Autodesk Inventor part; units mm, degrees
ref_plane "YZ Plane" through (0, 0, 0) normal (1, 0, 0) x (0, 1, 0)
ref_plane "XZ Plane" through (0, 0, 0) normal (0, 1, 0) x (-1, 0, 0)
ref_plane "XY Plane" through (0, 0, 0) normal (0, 0, 1) x (1, 0, 0)
sketch "Sketch1" plane through (0, 0, 0) normal (1, 0, 0) x (0, 1, 0)
  line L0 (0, 0) -> (20.7, 0)
  line L1 (20.7, 0) -> (20.7, -45.6)
  line L2 (20.7, -45.6) -> (0, -45.6)
  line L3 (0, -45.6) -> (0, 0)
  circle A0 centre (10.35, -9.5) radius 8
  circle A1 centre (10.35, -35.5) radius 8
  line L4 (21.7, -46.6) -> (21.7, 1)
  line L5 (21.7, 1) -> (-1, 1)
  line L6 (-1, 1) -> (-1, -46.6)
  line L7 (-1, -46.6) -> (21.7, -46.6)
  dimension "Breite" = 20.7
  dimension "Länge" = 45.6
  dimension "Kreise1" = 16
  dimension "BreiteBisKreise1" = 9.5
  dimension "LangeBisKreise" = 10.35
  dimension "KreiseCenter1BisKreiseCenter2" = 26
  dimension "Kreise2" = 16
  dimension "LangeBisKreise2" = 10.35
  dimension "d14" = 1
extrude "Extrusion1" add sketch "Sketch1" along normal blind 15 contours L0 L1 L2 L3 | A0 | A1
extrude "Extrusion2" add sketch "Sketch1" along normal up to surface (15 mm away) contours L7 L6 L5 L4
sketch "Sketch2" plane through (15, 0, 0) normal (1, 0, 0) x (0, 0, -1)
  line L0 (0, 20.7) -> (45.6, 20.7)
  line L1 (56.12, 0) -> (-10.52, 0)
  line L2 (45.6, 20.7) -> (45.6, 0)
  line L3 (0, -5.54) -> (0, 26.24)
  line L4 (0, 20.7) -> (45.6, 20.7)
  line L5 (45.6, 20.7) -> (45.6, 0)
  line L6 (45.6, 0) -> (0, 0)
  line L7 (0, 0) -> (0, 20.7)
extrude "Extrusion3" cut sketch "Sketch2" against normal blind 13
extrude "Extrusion4" cut sketch "Sketch1" along normal blind 11 contours A0 | A1
sketch "Sketch3" plane through (15, 0, 0) normal (1, 0, 0) x (0, 0, -1)
  line L0 (45.6, 20.7) -> (45.6, 0)
  line L1 (45.6, 0) -> (0, 0)
  line L2 (0, 0) -> (0, 20.7)
  line L3 (0, 20.7) -> (45.6, 20.7)
  line L4 (-1, 21.7) -> (46.6, 21.7)
  line L5 (-1, -1) -> (-1, 21.7)
  line L6 (46.6, -1) -> (-1, -1)
  line L7 (46.6, 21.7) -> (46.6, -1)
  line L8 (0, 0) -> (0, 20.7)
  line L9 (0, 0) -> (16.5, 0)
  line L10 (45.6, 0) -> (0, 0)
  line L11 (45.6, 20.7) -> (45.6, 0)
  line L12 (45.6, 0) -> (29.1, 0)
  line L13 (-1, -1) -> (46.6, -1)
  line L14 (16.5, -1) -> (16.5, -10.5)
  line L15 (29.1, -1) -> (29.1, -10.5)
  line L16 (16.5, -10.5) -> (29.1, -10.5)
  dimension "d21" = 16.5
  dimension "d22" = 16.5
  dimension "d23" = 9.5
  dimension "d24" = 1
  dimension "d26" = 12.6
extrude "Extrusion5" add sketch "Sketch3" against normal blind 4 contours L6 L15 L16 L14
sketch "Sketch4" plane through (15, 0, 0) normal (1, 0, 0) x (0, 0, -1)
  line L0 (45.6, 20.7) -> (45.6, 0)
  line L1 (45.6, 0) -> (0, 0)
  line L2 (0, 0) -> (0, 20.7)
  line L3 (0, 20.7) -> (45.6, 20.7)
  line L4 (-1, 21.7) -> (46.6, 21.7)
  line L5 (-1, -1) -> (-1, 21.7)
  line L6 (16.5, -1) -> (-1, -1)
  line L7 (16.5, -1) -> (16.5, -10.5)
  line L8 (16.5, -10.5) -> (29.1, -10.5)
  line L9 (29.1, -10.5) -> (29.1, -1)
  line L10 (46.6, -1) -> (29.1, -1)
  line L11 (46.6, 21.7) -> (46.6, -1)
  line L12 (29.1, -10.5) -> (29.1, -1)
  line L13 (29.1, -10.5) -> (16.5, -10.5)
  line L14 (29.1, -1) -> (16.5, -1)
  line L15 (16.5, -1) -> (16.5, -10.5)
  line L16 (16.5, -10.5) -> (29.1, -10.5)
  line L17 (29.1, -10.5) -> (29.1, -1)
  line L18 (17, -1.5) -> (28.6, -1.5)
  line L19 (28.6, -1.5) -> (28.6, -10)
  line L20 (28.6, -10) -> (17, -10)
  line L21 (17, -10) -> (17, -1.5)
  line L22 (17, -1.5) -> (17, 0)
  line L23 (45.6, 0) -> (0, 0)
  line L24 (28.6, -1.5) -> (28.6, 0)
  line L25 (17, 0) -> (28.6, 0)
  line L26 (17, -10) -> (17, -10.5)
  line L27 (28.6, -10) -> (28.6, -10.5)
  dimension "d29" = 0.5
extrude "Extrusion6" cut sketch "Sketch4" against normal blind 1 contours L24 L14 L22 L1 | L24 L18 L22 L14 | L19 L20 L21 L18 | L27 L8 L26 L20
fillet "Fillet1" radius 2 2 edges at (13, -1, -29.1) (13, -1, -16.5)
fillet "Fillet2" radius 2 4 edges at (7.5, -1, 1) (7.5, -1, -46.6) (7.5, 21.7, -46.6) (7.5, 21.7, 1)
fillet "Fillet3" radius 1 1 edges at (14, -10.5, -22.8)
fillet "Fillet4" radius 1 2 edges at (13, -10.5, -29.1) (13, -10.5, -16.5)
properties part number "Ultaschal Sensor Gehäuse"
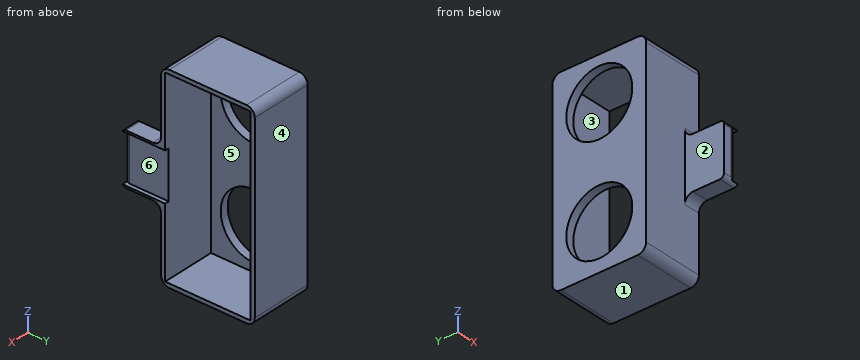
Geometry: final body of the model. Coordinates: model frame, mm. Face numbers are marked on the shaded views. A direction names the side the tool comes from. Give positions to 0.01 mm unless a question says otherwise; leave off trailing zeros. Write each loop counter-clockwise with the first axis right and the second up, starting at its lowest first coordinate (ties: lowest second). Pieces come first, ordered by that corner, then holes. Notation, with made-up numbers: (-26.75, 32) -> (32.25, 32) arc R25 cw to (32.25, 64) -> close; hole circle Ø10 at (22.5, -37.5). An arc over 180 degrees is marked (long way). Answer in a Markdown table with one row per item.
(1) Ray query, line 1 along Z through (x, y) = (1.15, 10.35); line 2 along Y through (x, z) = (0.6, -9.5); line 3 along Z through (x, y) = (13.75, 13.5). Return the intervals inside material, ascending. Write a range as [from, to].
Answers below:
| item | result |
|---|---|
| line 1 | [-46.6, -43.5], [-27.5, -17.5], [-1.5, 1] |
| line 2 | [-1, 2.35], [18.35, 21.7] |
| line 3 | [-46.6, -45.6], [0, 1] |
(2) Section query C-C on x = 10.25. Return loops of the section in (y, z), then the cut area to 3 significant figures.
Answers below:
| item | result |
|---|---|
| outline | (-1, -44.6) arc R2 ccw to (1, -46.6) -> (19.7, -46.6) arc R2 ccw to (21.7, -44.6) -> (21.7, -1) arc R2 ccw to (19.7, 1) -> (1, 1) arc R2 ccw to (-1, -1) -> close; hole (0, -45.6) -> (20.7, -45.6) -> (20.7, 0) -> (0, 0) -> close |
| area | 133 mm^2 |
(3) Section query A-A on z = -35.5. Return loops of the section in (x, y), then the cut area to 3 significant figures.
Answers below:
| item | result |
|---|---|
| outline | (0, -1) -> (15, -1) -> (15, 0) -> (2, 0) -> (2, 2.35) -> (0, 2.35) -> close; (0, 18.35) -> (2, 18.35) -> (2, 20.7) -> (15, 20.7) -> (15, 21.7) -> (0, 21.7) -> close |
| area | 39.4 mm^2 |
(4) Section query D-D on z = -21. Return loops of the section in (x, y), then the cut area to 3 significant figures.
Answers below:
| item | result |
|---|---|
| outline | (0, -1) -> (11, -1) -> (11, -10.5) -> (13, -10.5) arc R1 ccw to (14, -9.5) -> (14, 0) -> (2, 0) -> (2, 20.7) -> (15, 20.7) -> (15, 21.7) -> (0, 21.7) -> close |
| area | 98.7 mm^2 |
(5) Set-up query: the marked faces 4, 5 and 6. Return all of +Z, -Z, +X, -X, +Y, -Y with unobstructed straight access to the full face (end or side cutting, diameter ignored); none if empty.
Answers below:
| item | result |
|---|---|
| face 4 | +Z, -Z, +X, -X, +Y |
| face 5 | +X |
| face 6 | +X, -Y |
(6) Section query B-B on y = 10.35. Return loops of the section in (x, z).
Answers below:
| item | result |
|---|---|
| outline | (0, -46.6) -> (15, -46.6) -> (15, -45.6) -> (2, -45.6) -> (2, -43.5) -> (0, -43.5) -> close; (0, -27.5) -> (2, -27.5) -> (2, -17.5) -> (0, -17.5) -> close; (0, -1.5) -> (2, -1.5) -> (2, 0) -> (15, 0) -> (15, 1) -> (0, 1) -> close |
(7) Pin query (flat end, axial travel): pin 1 (7.5 mm diameter, centred on x = 6.5, z = -24.5, fed in from -Y); pin 2 (4.5 mm diameter, centred on x = 12.5, y = -5, fed in from +Z); pin 3 (6 mm diameter, centred on x = 11, y = -5.5, fed in from +Z); pin 4 (12 mm diameter, centred on y = 7, z = -19, fed in from -X). Return the tip coordinate at first contact, or that it passes through.
Answers below:
| item | result |
|---|---|
| pin 1 | y = -1 |
| pin 2 | z = -16.48 |
| pin 3 | z = -16.44 |
| pin 4 | x = 0 |
(8) Draft query along Z for the marked faces 1, 2 and 3. Return one class per face: +Z half, -Z half, draft (parallel to the pull), parting line (faces both ways), or undercut.
Answers below:
| item | result |
|---|---|
| face 1 | -Z half |
| face 2 | draft |
| face 3 | undercut |
